Autodesk Inventor part; units mm, degrees
ref_plane "YZ Plane" through (0, 0, 0) normal (1, 0, 0) x (0, 1, 0)
ref_plane "XZ Plane" through (0, 0, 0) normal (0, 1, 0) x (-1, 0, 0)
ref_plane "XY Plane" through (0, 0, 0) normal (0, 0, 1) x (1, 0, 0)
sketch "Sketch1" plane through (0, 0, 0) normal (0, 0, 1) x (1, 0, 0)
  line L0 (0, 0) -> (19, 0)
  line L1 (19, 0) -> (19, 22)
  line L2 (19, 22) -> (0, 22)
  line L3 (0, 22) -> (0, 0)
  dimension "d0" = 19
  dimension "d1" = 22
extrude "Extrusion1" add sketch "Sketch1" along normal blind 1
sketch "Sketch2" plane through (0, 0, 1) normal (0, 0, 1) x (1, 0, 0)
  line L0 (0, 0) -> (19, 0)
  line L1 (0, 0) -> (2.9, 0)
  line L2 (2.9, 0) -> (2.9, 12)
  line L3 (2.9, 12) -> (0, 12)
  line L4 (0, 12) -> (0, 0)
  line L5 (2.9, 12) -> (15.9, 12)
  line L6 (15.9, 12) -> (15.9, -2)
  line L7 (15.9, -2) -> (2.9, -2)
  line L8 (2.9, -2) -> (2.9, 12)
  dimension "d4" = 2.9
  dimension "d5" = 12
  dimension "d6" = 13
  dimension "d7" = 14
extrude "Extrusion2" add sketch "Sketch2" along normal blind 7 contours L2 L5 L6 L0 | L0 L6 L7 L8
sketch "Sketch3" plane through (0, 0, 0) normal (0, 0, -1) x (-1, 0, 0)
  line L0 (-19, 0) -> (-19, 22)
  line L1 (-19, 0) -> (-13.5, 0)
  line L2 (-13.5, 0) -> (-13.5, 5)
  line L3 (-13.5, 5) -> (-19, 5)
  line L4 (-19, 5) -> (-19, 0)
  line L5 (-13.5, 0) -> (-5.5, 0)
  line L6 (-5.5, 0) -> (-5.5, 5.5)
  line L7 (-5.5, 5.5) -> (-13.5, 5.5)
  line L8 (-13.5, 5.5) -> (-13.5, 0)
  line L9 (-13.5, 0) -> (-5.5, 0)
  line L10 (-5.5, 0) -> (-5.5, -1.5)
  line L11 (-5.5, -1.5) -> (-13.5, -1.5)
  line L12 (-13.5, -1.5) -> (-13.5, 0)
  point P0 (0, 0)
  dimension "d10" = 5.5
  dimension "d11" = 5
  dimension "d12" = 8
  dimension "d13" = 5.5
  dimension "d16" = 8
  dimension "d17" = 1.5
extrude "Extrusion3" add sketch "Sketch3" along normal blind 3 contours L2 L8 L7 L6 L5 | L5 L10 L11 L12
sketch "Sketch4" plane through (0, 0, 1) normal (0, 0, 1) x (1, 0, 0)
  line L0 (19, 22) -> (0, 22)
  line L1 (0, 22) -> (1.5, 22)
  line L2 (1.5, 22) -> (1.5, 20.5)
  line L3 (1.5, 20.5) -> (0, 20.5)
  line L4 (0, 20.5) -> (0, 22)
  line L5 (19, 22) -> (17.5, 22)
  line L6 (17.5, 22) -> (17.5, 20.5)
  line L7 (17.5, 20.5) -> (19, 20.5)
  line L8 (19, 20.5) -> (19, 22)
  line L9 (17.5, 20.5) -> (1.5, 20.5)
  line L10 (1.5, 20.5) -> (1.5, 13.5)
  line L11 (1.5, 13.5) -> (17.5, 13.5)
  line L12 (17.5, 13.5) -> (17.5, 20.5)
  point P0 (0, 0)
  dimension "d18" = 1.5
  dimension "d19" = 1.5
  dimension "d20" = 1.5
  dimension "d21" = 1.5
  dimension "d22" = 16
  dimension "d23" = 7
extrude "Extrusion4" add sketch "Sketch4" along normal blind 3 contours L12 L11 L10 L9
sketch "Sketch5" plane through (0, 0, 4) normal (0, 0, 1) x (1, 0, 0)
  line L0 (17.5, 20.5) -> (1.5, 20.5)
  line L1 (17.5, 20.5) -> (12.5, 20.5)
  line L2 (12.5, 20.5) -> (12.5, 15.5)
  line L3 (12.5, 15.5) -> (17.5, 15.5)
  line L4 (17.5, 15.5) -> (17.5, 20.5)
  point P0 (0, 0)
  dimension "d26" = 5
  dimension "d27" = 5
extrude "Extrusion5" add sketch "Sketch5" along normal blind 2
sketch "Sketch6" plane through (1.5, 20.5, 1) normal (0, 1, 0) x (1, 0, 0)
  line L0 (0, -3) -> (16, -3)
  line L1 (0, -3) -> (11, -3)
  line L2 (11, -3) -> (11, 0)
  line L3 (11, 0) -> (0, 0)
  line L4 (0, 0) -> (0, -3)
  point P0 (-1.5, 1)
  dimension "d30" = 11
  dimension "d31" = 3
extrude "Extrusion6" cut sketch "Sketch6" against normal blind 0.5
sketch "Sketch7" plane through (17.5, 13.5, 1) normal (1, 0, 0) x (0, 0, -1)
  line L0 (0, 0) -> (-3, 0)
  line L1 (-3, 0) -> (0, 0)
  line L2 (0, 0) -> (0, 2)
  line L3 (0, 2) -> (-3, 2)
  line L4 (-3, 2) -> (-3, 0)
  point P0 (1, -13.5)
  dimension "d34" = 3
  dimension "d35" = 2
extrude "Extrusion7" cut sketch "Sketch7" against normal blind 0.5
sketch "Sketch8" plane through (0, 0, 0) normal (0, 0, -1) x (-1, 0, 0)
  line L0 (-19, 0) -> (-19, 22)
  line L1 (-19, 0) -> (-18, 0)
  line L2 (-18, 0) -> (-18, 6)
  line L3 (-18, 6) -> (-19, 6)
  line L4 (-19, 6) -> (-19, 0)
  line L5 (-18, 6) -> (-16.75, 6)
  line L6 (-16.75, 6) -> (-16.75, 5.5)
  line L7 (-16.75, 5.5) -> (-18, 5.5)
  line L8 (-18, 5.5) -> (-18, 6)
  line L9 (-16.75, 5.5) -> (-15.75, 5.5)
  line L10 (-15.75, 5.5) -> (-15.75, 6)
  line L11 (-15.75, 6) -> (-16.75, 6)
  line L12 (-16.75, 6) -> (-16.75, 5.5)
  line L13 (-15.75, 5.5) -> (-14.5, 5.5)
  line L14 (-14.5, 5.5) -> (-14.5, 6)
  line L15 (-14.5, 6) -> (-15.75, 6)
  line L16 (-15.75, 6) -> (-15.75, 5.5)
  line L17 (-13.5, 5.5) -> (-5.5, 5.5)
  line L18 (-14.5, 6) -> (-13.5, 6)
  line L19 (-13.5, 6) -> (-13.5, 5.5)
  line L20 (-13.5, 5.5) -> (-14.5, 5.5)
  line L21 (-14.5, 5.5) -> (-14.5, 6)
  point P0 (0, 0)
  dimension "d38" = 1
  dimension "d39" = 6
  dimension "d40" = 1.25
  dimension "d41" = 0.5
  dimension "d42" = 1
  dimension "d43" = 1.25
  dimension "d44" = 1
  dimension "d45" = 0.5
extrude "Extrusion8" add sketch "Sketch8" along normal blind 1.5 contours L5 L6 L7 L2 | L15 L14 L13 L10
sketch "Sketch9" plane through (14.5, 6, 0) normal (0, 1, 0) x (1, 0, 0)
  line L0 (1.25, 1.5) -> (0, 1.5)
  line L1 (0, 1.5) -> (1.25, 1.5)
  line L2 (1.25, 1.5) -> (1.25, 0)
  line L3 (1.25, 0) -> (0, 0)
  line L4 (0, 0) -> (0, 1.5)
  line L5 (3.5, 1.5) -> (2.25, 1.5)
  line L6 (2.25, 1.5) -> (3.5, 1.5)
  line L7 (3.5, 1.5) -> (3.5, 0)
  line L8 (3.5, 0) -> (2.25, 0)
  line L9 (2.25, 0) -> (2.25, 1.5)
  point P0 (-14.5, 0)
  dimension "d48" = 1.25
  dimension "d49" = 1.5
  dimension "d50" = 1.25
  dimension "d51" = 1.5
extrude "Extrusion9" add sketch "Sketch9" along normal blind 0.5
sketch "Sketch10" plane through (16.75, 5.5, 0) normal (0, -1, 0) x (1, 0, 0)
  line L0 (1.25, 0) -> (1.25, -1.5)
  line L1 (1.25, -1.5) -> (0.625, -1.5)
  line L2 (0.625, -1.5) -> (0.625, -0.875)
  line L3 (0.625, -0.875) -> (1.25, -0.875)
  line L4 (1.25, -0.875) -> (1.25, -1.5)
  circle A0 centre (0.625, -0.875) radius 0.5
  line L5 (-1, -1.5) -> (-2.25, -1.5)
  line L6 (-1, -1.5) -> (-1.625, -1.5)
  line L7 (-1.625, -1.5) -> (-1.625, -0.875)
  line L8 (-1.625, -0.875) -> (-1, -0.875)
  line L9 (-1, -0.875) -> (-1, -1.5)
  circle A1 centre (-1.625, -0.875) radius 0.5
  point P0 (-16.75, 0)
  dimension "d54" = 0.625
  dimension "d55" = 0.625
  dimension "d56" = 1
  dimension "d57" = 0.625
  dimension "d58" = 0.625
  dimension "d59" = 1
extrude "Extrusion10" add sketch "Sketch10" along normal blind 3.5 contours A0 L2 L3 | L3 L2 A0 | A1 L8 L7 | L7 L8 A1
sketch "Sketch11" plane through (17.375, 2, -0.875) normal (0, -1, 0) x (1, 0, 0)
  circle A0 centre (0, 0) radius 0.625
  point P0 (-17.375, 0.875)
  dimension "d62" = 1.25
extrude "Extrusion11" add sketch "Sketch11" along normal blind 5.25
sketch "Sketch12" plane through (0, 0, 0) normal (0, 0, -1) x (-1, 0, 0)
  point P0 (0, 0)
sketch "Sketch13" plane through (0, 0, 0) normal (0, 0, -1) x (-1, 0, 0)
  line L0 (0, 0) -> (-2.9, 0)
  line L1 (0, 0) -> (-1, 0)
  line L2 (-1, 0) -> (-1, 6.5)
  line L3 (-1, 6.5) -> (0, 6.5)
  line L4 (0, 6.5) -> (0, 0)
  line L5 (-1, 6.5) -> (-2.25, 6.5)
  line L6 (-2.25, 6.5) -> (-2.25, 5.5)
  line L7 (-2.25, 5.5) -> (-1, 5.5)
  line L8 (-1, 5.5) -> (-1, 6.5)
  line L9 (-2.25, 6.5) -> (-3.25, 6.5)
  line L10 (-3.25, 6.5) -> (-3.25, 5.5)
  line L11 (-3.25, 5.5) -> (-2.25, 5.5)
  line L12 (-2.25, 5.5) -> (-2.25, 6.5)
  line L13 (-3.25, 6.5) -> (-4.5, 6.5)
  line L14 (-4.5, 6.5) -> (-4.5, 5.5)
  line L15 (-4.5, 5.5) -> (-3.25, 5.5)
  line L16 (-3.25, 5.5) -> (-3.25, 6.5)
  dimension "d65" = 1
  dimension "d66" = 6.5
  dimension "d67" = 1.25
  dimension "d68" = 1
  dimension "d69" = 1
  dimension "d70" = 1
  dimension "d71" = 1.25
  dimension "d72" = 1
extrude "Extrusion12" add sketch "Sketch13" along normal blind 1.5 contours L7 L6 L5 L2 | L15 L14 L13 L10
sketch "Sketch14" plane through (3.25, 5.5, 0) normal (0, -1, 0) x (1, 0, 0)
  line L0 (0, -1.5) -> (1.25, -1.5)
  line L1 (1.25, -1.5) -> (0.625, -1.5)
  line L2 (0.625, -1.5) -> (0.625, -0.875)
  line L3 (0.625, -0.875) -> (1.25, -0.875)
  line L4 (1.25, -0.875) -> (1.25, -1.5)
  circle A0 centre (0.625, -0.875) radius 0.5
  line L5 (-2.25, -1.5) -> (-1, -1.5)
  line L6 (-1, -1.5) -> (-1.625, -1.5)
  line L7 (-1.625, -1.5) -> (-1.625, -0.875)
  line L8 (-1.625, -0.875) -> (-1, -0.875)
  line L9 (-1, -0.875) -> (-1, -1.5)
  circle A1 centre (-1.625, -0.875) radius 0.5
  point P0 (-3.25, 0)
  dimension "d75" = 0.625
  dimension "d76" = 0.625
  dimension "d77" = 1
  dimension "d78" = 0.625
  dimension "d79" = 0.625
  dimension "d80" = 1
extrude "Extrusion13" add sketch "Sketch14" along normal blind 3.5 contours A0 L3 L2 | L2 L3 A0 | A1 L8 L7 | L7 L8 A1
sketch "Sketch15" plane through (3.875, 2, -0.875) normal (0, -1, 0) x (1, 0, 0)
  circle A0 centre (0, 0) radius 0.625
  point P0 (-3.875, 0.875)
  dimension "d83" = 1.25
extrude "Extrusion14" add sketch "Sketch15" along normal blind 5.25
sketch "Sketch16" plane through (1.625, 2, -0.875) normal (0, -1, 0) x (1, 0, 0)
  circle A0 centre (0, 0) radius 0.625
  point P0 (-1.625, 0.875)
  dimension "d86" = 1.25
extrude "Extrusion15" add sketch "Sketch16" along normal blind 5.25
sketch "Sketch17" plane through (15.125, 2, -0.875) normal (0, -1, 0) x (1, 0, 0)
  circle A0 centre (0, 0) radius 0.625
  point P0 (-15.125, 0.875)
  dimension "d89" = 1.25
extrude "Extrusion16" add sketch "Sketch17" along normal blind 5.25
fillet "Fillet1" radius 0.5 4 edges at (16.75, -3.25, -0.875) (14.5, -3.25, -0.875) (3.25, -3.25, -0.875) (1, -3.25, -0.875)
sketch "Sketch18" plane through (2.9, -2, 1) normal (0, -1, 0) x (1, 0, 0)
  line L0 (0, 7) -> (13.0027, 7) construction
  line L1 (13.0027, 7) -> (13.0027, 1.5822) construction
  line L2 (13.0027, 1.5822) -> (0, 1.5822) construction
  line L3 (0, 1.5822) -> (0, 7) construction
  point P0 (-2.9, -1)
sketch "Sketch19" plane through (5.5, -1.5, 0) normal (0, -1, 0) x (1, 0, 0)
  line L0 (8, 0) -> (0, 0)
  line L1 (0, 0) -> (8, 0) construction
  line L2 (8, 0) -> (8, -3.25) construction
  line L3 (8, -3.25) -> (0, -3.25) construction
  line L4 (0, -3.25) -> (0, 0) construction
  point P0 (-5.5, 0)
properties part number "Battery-Management"
Source: CAD feature listing. Evaluate the final solid. Frame: model axes, mm. A direction names the side the tool comes from. Round coordinates to 2 decimals unless told otherwise and drop trailing zeros. Order: outer loops, then holes, each group sorted by start corner. A loop starts at its lowest first (then second) coordinate and runs counter-clockwise, first axis right, second up. Notation, with made-up numbers: (60, -39) -> (87, -39) arc R19 ccw to (87, -29) -> close; hole circle Ø11 at (10, 76.5). An arc over 180 degrees is marked (long way). One line per item, written item: value. Start each with the question number.
Q1. Section query B-B (x = 10.5). Return the cut outline in (y, z), plus the area to 4 significant figures.
Q2. Section query A-A (z = 2). Return the cut outline in (x, y).
Q3. Pin query (flat end, axial travel): pin 1 (1.6 mm diameter, centred on y = 15, z = 3, fed in from +X); pin 2 (5 mm diameter, centred on x = 8, z = 5, fed in from -Y); pin 3 (0.6 mm diameter, centred on x = 17.5, z = -1, fed in from +Y); pin 4 (1.4 mm diameter, centred on x = 17.5, z = -0.5, fed in from +Y). Return the tip coordinate at first contact, or that it passes through.
Q4. Material intervals for probe 1 along Y at (x, z) = (13, 4.75); probe 2 along Y at (x, z) = (10.25, 3.5); probe 3 along Y at (x, z) = (15.5, 6.5), sorted ascending.
Q5. Section query D-D (y = 3.75). Return the cut outline in (x, z) (3 decimals).
Q6. Access query for faces 5 (the cylindrical face through (17.85, 3.77, -1.03)), 6 (the flat face through (9, -1, 1)), 7 (the flat face through (15, 18, 6)). Directions: +Z, -Z, +X, -X, +Y, -Y. A direction counts if a zero-diameter tool reaches every point of the face in a straight line with its end or side. Return the directions, or none.
Q7. Draft query along X for faces 1 (the cylindrical face through (3.375, 3.774, -0.897)), 2 (the flat face through (17, 15, 3)), 3 (the cylindrical face through (2.22, -0.34, -1.06)), 4 (the flat face through (2, 6.5, -1)). Return one class per face: pulls with the +X half, pulls with the -X half, needs draft (parallel to the pull), parting line crosses it, or undercut.
Q8. Section query C-C (z = 4.5). Return the cut outline in (x, y).
Findings below:
1. outline: (-2, 1) -> (0, 1) -> (0, 0) -> (-1.5, 0) -> (-1.5, -3) -> (5.5, -3) -> (5.5, 0) -> (22, 0) -> (22, 1) -> (20, 1) -> (20, 4) -> (13.5, 4) -> (13.5, 1) -> (12, 1) -> (12, 8) -> (-2, 8) -> close
1. area: 160.5 mm²
2. outline: (1.5, 13.5) -> (17, 13.5) -> (17, 15.5) -> (17.5, 15.5) -> (17.5, 20.5) -> (12.5, 20.5) -> (12.5, 20) -> (1.5, 20) -> close; (2.9, -2) -> (15.9, -2) -> (15.9, 12) -> (2.9, 12) -> close
3. pin 1: x = 17.5
3. pin 2: y = -2
3. pin 3: y = 6.5
3. pin 4: y = 22
4. probe 1: -2 to 12, 15.5 to 20.5
4. probe 2: -2 to 12, 13.5 to 20
4. probe 3: -2 to 12
5. outline: (0, 0) -> (5.5, 0) -> (5.5, -3) -> (13.5, -3) -> (13.5, 0) -> (19, 0) -> (19, 1) -> (15.9, 1) -> (15.9, 8) -> (2.9, 8) -> (2.9, 1) -> (0, 1) -> close; circle Ø1 at (1.625, -0.875); circle Ø1 at (3.875, -0.875); circle Ø1 at (15.125, -0.875); circle Ø1 at (17.375, -0.875)
6. face 5: none
6. face 6: +X, -X, -Y
6. face 7: +Z, +X, -X, +Y
7. face 1: undercut
7. face 2: pulls with the +X half
7. face 3: undercut
7. face 4: needs draft
8. outline: (2.9, -2) -> (15.9, -2) -> (15.9, 12) -> (2.9, 12) -> close; (12.5, 15.5) -> (17.5, 15.5) -> (17.5, 20.5) -> (12.5, 20.5) -> close
